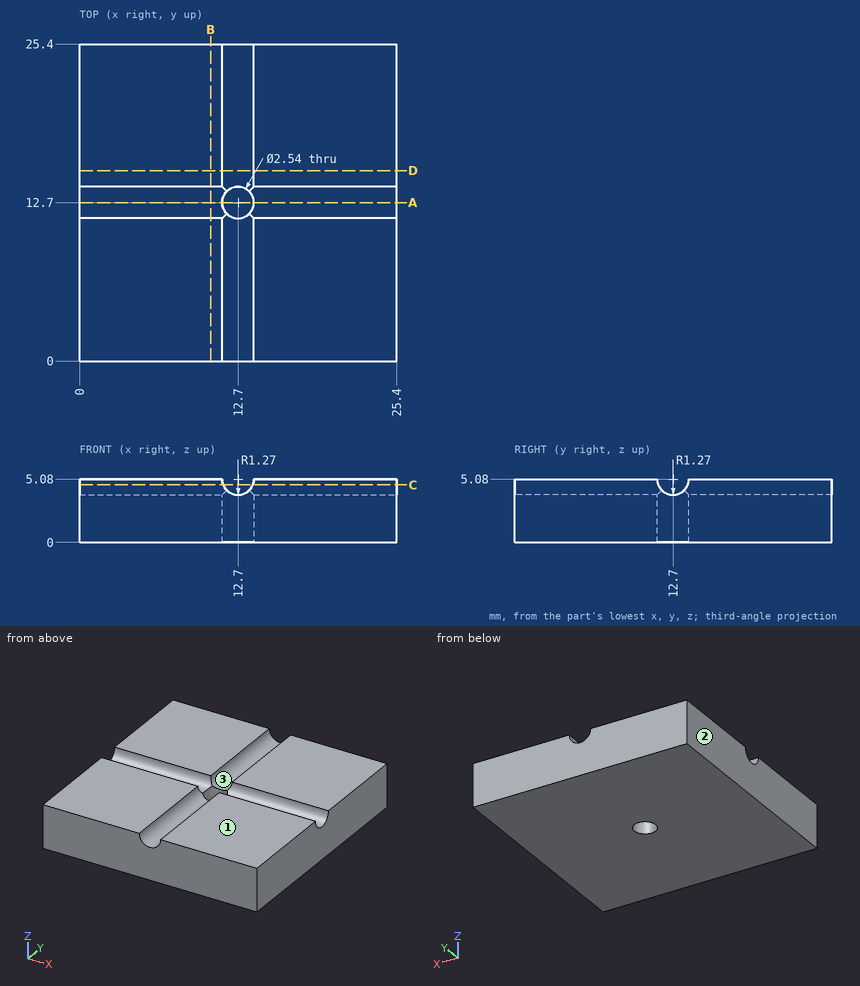
The figure shows three views and two pictorial views of one solid part (mm, origin at its lowest corner). Answer the questions. Round coordinates to 2 decimals unless told otherwise and drop trailing zeros. Write each loop counter-clockwise with the first axis right and the second up, starting at its lowest first coordinate (ties: lowest second). Pieces come first, ordered by that corner, then holes. Notation, with made-up numbers: (-10, 77) - (49, 77) arc R11 cw to (49, 84) - close; hole circle Ø3 at (-10.5, 75). An arc over 180 degrees is marked (long way). Answer in a Markdown table with one row per item. Add a question column.
1. A cutting plane is placed at B-B, the plane x = 10.5. Determine the outline of the cut face in (y, z).
2. Given pin 1 (3 mm diameter, centred on x = 12.7, y = 12.7, fed in from -Z), flat-ended and moving along its own axis, determine where the tip first touches the part or whether it passes through.
3. A cutting plane is placed at A-A, the plane y = 12.7. Determine the outline of the cut face in (x, z), and give its area (3 significant figures).
4. Find the intervals of material crossed by line 1 along X through (y, z) = (12.7, 2.2); line 2 along X through (y, z) = (15, 4), in increasing order. Write a range as from..to.
5. The mould has two halves that part along X. Classify the marked faces 1, 2 and 3: +X half, -X half, draft (parallel to the pull), parting line (faces both ways), or undercut.
6. A cutting plane is placed at C-C, the plane z = 4.6. Determine the outline of the cut face in (x, y), and give its area (3 significant figures).
Worked out:
| question | item | result |
|---|---|---|
| 1 | outline | (0, 0) - (25.4, 0) - (25.4, 5.08) - (13.97, 5.08) arc R1.27 cw to (11.43, 5.08) - (0, 5.08) - close |
| 2 | pin 1 | z = 0 |
| 3 | outline | (0, 0) - (11.43, 0) - (11.43, 3.81) - (0, 3.81) - close; (13.97, 0) - (25.4, 0) - (25.4, 3.81) - (13.97, 3.81) - close |
| 3 | area | 87.1 mm^2 |
| 4 | line 1 | 0..11.43, 13.97..25.4 |
| 4 | line 2 | 0..12.03, 13.37..25.4 |
| 5 | face 1 | draft |
| 5 | face 2 | -X half |
| 5 | face 3 | undercut |
| 6 | outline | (0, 0) - (11.52, 0) - (11.52, 11.52) - (0, 11.52) - close; (0, 13.88) - (11.52, 13.88) - (11.52, 25.4) - (0, 25.4) - close; (13.88, 0) - (25.4, 0) - (25.4, 11.52) - (13.88, 11.52) - close; (13.88, 13.88) - (25.4, 13.88) - (25.4, 25.4) - (13.88, 25.4) - close |
| 6 | area | 531 mm^2 |
